Geometry check sheet. Reference: drawing and pictorial views, mm from the part's lowest x, y, z. Give positions to 0.01 mm unless a question says otherwise; leave off trailing zeros. Loops run counter-clockwise (first coordinate to the right, second up) from the corner with the lowest first, then second, coordinate; pieces in that order, holes last. Notation, with made-up numbers: (45, -14) -> (58, -14) arc R33 ccw to (58, 22) -> close; hole circle Ø7 at (3.5, 14.25). An arc over 180 degrees is marked (long way). Answer in a Markdown table with one row per item. Add a question column.
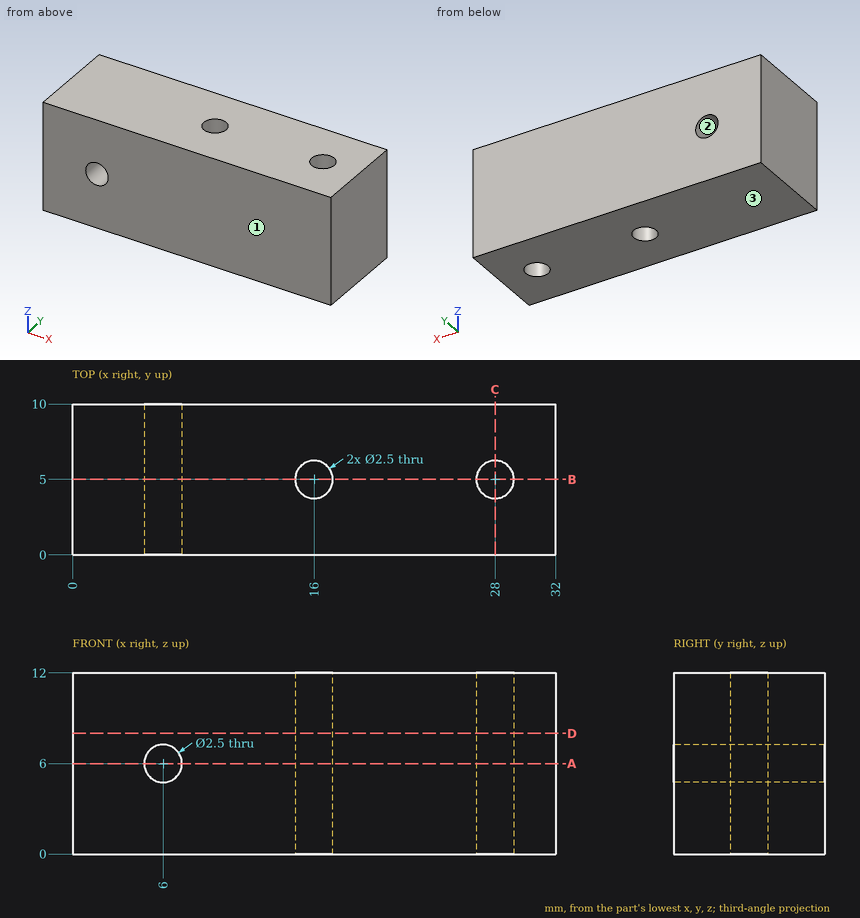
1. Sectioned sample at C-C (x = 28). Enter the section's corners in (y, z).
2. Sectioned sample at D-D (z = 8). Enter the section's corners in (x, y).
3. Release check for a two-part mould opening along Z. For the marked faces 1, 2 and 3 record: released by +Z, released by -Z, zero draft, split by the parting line, or undercut.
4. Material ranges on L1, parallel to Y at x = 28, z = 6.5; L2, parallel to Z at x = 6, y = 7.25; L3, parallel to X at y = 5.25, z = 6, recorded low to high. Write a range as from..to.
5. Sectioned sample at B-B (y = 5). Enter the section's corners in (x, z), plus the area to 3 significant figures.
6. Sectioned sample at A-A (z = 6). Enter the section's corners in (x, y), plus the area to 3 significant figures.
Response:
| question | item | result |
|---|---|---|
| 1 | outline | (0, 0) -> (3.75, 0) -> (3.75, 12) -> (0, 12) -> close; (6.25, 0) -> (10, 0) -> (10, 12) -> (6.25, 12) -> close |
| 2 | outline | (0, 0) -> (32, 0) -> (32, 10) -> (0, 10) -> close; hole circle Ø2.5 at (16, 5); hole circle Ø2.5 at (28, 5) |
| 3 | face 1 | zero draft |
| 3 | face 2 | undercut |
| 3 | face 3 | released by -Z |
| 4 | L1 | y = 0..3.75, 6.25..10 |
| 4 | L2 | z = 0..4.75, 7.25..12 |
| 4 | L3 | x = 0..4.75, 7.25..14.78, 17.22..26.78, 29.22..32 |
| 5 | outline | (0, 0) -> (14.75, 0) -> (14.75, 12) -> (0, 12) -> close; (17.25, 0) -> (26.75, 0) -> (26.75, 12) -> (17.25, 12) -> close; (29.25, 0) -> (32, 0) -> (32, 12) -> (29.25, 12) -> close; hole circle Ø2.5 at (6, 6) |
| 5 | area | 319 mm2 |
| 6 | outline | (0, 0) -> (4.75, 0) -> (4.75, 10) -> (0, 10) -> close; (7.25, 0) -> (32, 0) -> (32, 10) -> (7.25, 10) -> close; hole circle Ø2.5 at (16, 5); hole circle Ø2.5 at (28, 5) |
| 6 | area | 285 mm2 |
